Geometry check sheet. Reference: the model listing, model coordinates, mm. Face numbers are marked on the shaded views. A direction names the side the tool comes from. Give positions to 0.01 mm unless a question says otherwise; leave off trailing zeros. Write each loop counter-clockwise with the first axis right and the second up, starting at its lowest first coordinate (ties: lowest second). Pieces come first, ordered by that corner, then holes. Notation, with made-up numbers: (16.5, 68) - (60.5, 68) arc R22 ccw to (60.5, 80) - close; hole circle Ø11 at (-39, -8). An arc over 180 degrees is marked (long way). Use a Markdown table: item, result.
```python
from build123d import *

# Parameters (mm, degrees)
SKETCH1_R           = 11
BOSS_EXTRUDE1_DEPTH = 2
SKETCH2_R           = 9.5
BOSS_EXTRUDE2_DEPTH = 5
SKETCH3_R           = 5.5
BOSS_EXTRUDE3_DEPTH = 17
SKETCH4_R           = 4.8
CUT_EXTRUDE1_DEPTH  = 25
SKETCH5_R           = 8.8
CUT_EXTRUDE2_DEPTH  = 5.5
FILLET1_R           = 2
FILLET2_R           = 1
FILLET3_R           = 1


with BuildPart() as part:
    # Sketch1 → Boss-Extrude1 (new body)
    with BuildSketch(Plane.XY):
        Circle(SKETCH1_R)
    extrude(amount=BOSS_EXTRUDE1_DEPTH)

    # Sketch2 → Boss-Extrude2 (add)
    with BuildSketch(Plane(origin=(0, 0, 0), x_dir=(-1, 0, 0), z_dir=(0, 0, -1))):
        Circle(SKETCH2_R)
    extrude(amount=BOSS_EXTRUDE2_DEPTH)

    # Sketch3 → Boss-Extrude3 (add)
    with BuildSketch(Plane.XY.offset(2)):
        Circle(SKETCH3_R)
    extrude(amount=BOSS_EXTRUDE3_DEPTH)

    # Sketch4 → Cut-Extrude1 (cut)
    with BuildSketch(Plane.XY.offset(19)):
        Circle(SKETCH4_R)
    extrude(amount=-CUT_EXTRUDE1_DEPTH, mode=Mode.SUBTRACT)

    # Sketch5 → Cut-Extrude2 (cut)
    with BuildSketch(Plane(origin=(0, 0, -5), x_dir=(-1, 0, 0), z_dir=(0, 0, -1))):
        Circle(SKETCH5_R)
    extrude(amount=-CUT_EXTRUDE2_DEPTH, mode=Mode.SUBTRACT)

    # Fillet1
    fillet1_edges = [part.edges().sort_by_distance(p)[0] for p in [
        (-4.8, 0, 0.5),
    ]]
    fillet(fillet1_edges, radius=FILLET1_R)

    # Fillet2
    fillet2_edges = [part.edges().sort_by_distance(p)[0] for p in [
        (-11, 0, 2),
    ]]
    fillet(fillet2_edges, radius=FILLET2_R)

    # Fillet3
    # the kernel refuses this fillet: 1 mm, written as the material it takes off along each edge
    with BuildSketch(Plane(origin=(0, 0, 19), x_dir=(1, 0, 0), z_dir=(0, -1, 0))) as fillet3_piece_1:
        with BuildLine():
            CenterArc((4.5, -0.953939201), FILLET3_R, 0, 72.542396876)
            Line((4.8, 0), (4.806, 0.019078784))
            ThreePointArc((4.806, 0.019078784), (5.15, 0.02), (5.5, 0.02))
            Line((5.5, 0.02), (5.52, 0))
            Line((5.52, 0), (5.52, -0.953939201))
            Line((5.52, -0.953939201), (5.5, -0.953939201))
        make_face()
    revolve(axis=Axis((0, 0, 19), (0, 0, 1)), mode=Mode.SUBTRACT)


solid = part.part
```
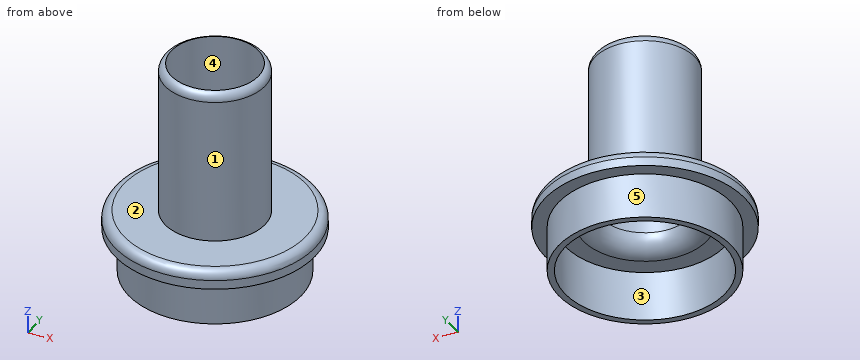
1) Section check A-A on y = 0. Record the boundary of the cut face in (x, z), then the cut area to 3 significant figures.
Working result:
| item | result |
|---|---|
| outline | (-11, 0) - (-9.5, 0) - (-9.5, -5) - (-8.8, -5) - (-8.8, 0.5) - (-6.8, 0.5) arc R2 ccw to (-4.8, 2.5) - (-4.8, 19) arc R1 ccw to (-5.5, 18.05) - (-5.5, 2) - (-10, 2) arc R1 ccw to (-11, 1) - close; (4.8, 2.5) arc R2 ccw to (6.8, 0.5) - (8.8, 0.5) - (8.8, -5) - (9.5, -5) - (9.5, 0) - (11, 0) - (11, 1) arc R1 ccw to (10, 2) - (5.5, 2) - (5.5, 18.05) arc R1 ccw to (4.8, 19) - close |
| area | 49.1 mm² |
2) Depth check by flat-ended pin: P1, Ø8, axis at x = 8.5, z = 12.5, coming from the +Y side; P2, Ø10.5, axis at x = 0, y = 0, coming from the -Z side; P3, Ø4, axis at y = 3.5, z = -0.5, coming from the +X side; P4, Ø5.5, axis at x = -1, y = -0.5, coming from the -Z side. Enter the tip coordinate at first touch or a pass-through.
Working result:
| item | result |
|---|---|
| P1 | stops at y = 3.16 |
| P2 | stops at z = 1.24 |
| P3 | stops at x = 10.89 |
| P4 | passes through |
3) Section check C-C on z = 10. Record the boundary of the cut face in (x, y).
Working result:
| item | result |
|---|---|
| outline | circle Ø11 at (0, 0); hole circle Ø9.6 at (0, 0) |
4) Mould release check, pull along X, two halves, no side actions. Record for the marked faces 1, 2 and 3: pulls with the +X half, pulls with the -X half, needs draft (parallel to the pull), parting line crosses it, or undercut.
Working result:
| item | result |
|---|---|
| face 1 | parting line crosses it |
| face 2 | needs draft |
| face 3 | undercut |
5) Set-up check for the marked faces 4 and 5: record each of +Z, -Z, +X, -X, +Y, -Y from which the full face is reachable in a straight line by a thin tool's end or side.
Working result:
| item | result |
|---|---|
| face 4 | +Z, -Z |
| face 5 | -Z |
6) Material ranges on L1, parallel to Y at x = 0, z = -2.8; L2, parallel to Y at x = 0, z = 8; L3, parallel to X at y = -3.5, z = -2, recorded low to high. Write a range as from..to.
Working result:
| item | result |
|---|---|
| L1 | y = -9.5..-8.8, 8.8..9.5 |
| L2 | y = -5.5..-4.8, 4.8..5.5 |
| L3 | x = -8.83..-8.07, 8.07..8.83 |
